from build123d import *

# Parameters (mm, degrees)
F1_DEPTH = 25.4
F2_SIZE  = 12.7
F3_T     = -2.54


with BuildPart() as f1:
    # F0 (on Top) → F1 (new body)
    with BuildSketch(Plane.XY):
        Polygon((4.5641, -68.949298), (57.429793, 38.427275), (-61.993893, 30.522022), align=None)
    extrude(amount=F1_DEPTH)

    # F2
    f2_edges = [f1.edges().sort_by_distance(p)[0] for p in [
        (30.996947, -15.261011, 25.4),
        (-28.714897, -19.213638, 25.4),
        (-2.28205, 34.474649, 25.4),
    ]]
    chamfer(f2_edges, length=F2_SIZE)

    # F3
    f3_openings = [f1.faces().sort_by_distance(p)[0] for p in [
        (0, 0, 25.4),
    ]]
    offset(amount=F3_T, openings=f3_openings)


solid = f1.part
Here's how the part is built. I have some questions about the finished solid (model axes, mm). A direction names the side the tool comes from. Coordinates: 2 decimals unless noted, no trailing zeros. Loops run counter-clockwise (first coordinate to the right, second up) from the corner with the lowest first, then second, coordinate; pieces in that order, holes last.
1. I need wall thicknesses on L1, parallel to Z at x = 2, y = -23.5; L2, parallel to X at y = -41, z = 14.75; L3, parallel to Y at x = -51.5, z = 2.75. Which ranges of each line are inside material? Lowest first, please.
2. For faces 1 (the flat face through (-0.879, 25.034, 18.62)), 2 (the flat face through (-1.021, 28.105, 19.139)), which set-ups out of +Z, -Z, +X, -X, +Y, -Y let a thin tool reach every point of the face, with its end or its side?
3. Imagine slicing it at D-D, the plane y = 10.5. Please give me the cut outline in (x, z), and give its area (3 significant figures).
4. Imagine slicing it at B-B, the plane x = 33. Please give me the cut outline in (y, z) (3 decimals), and give its area (3 significant figures).
5. For P1, Ø2, axis at x = -14.5, z = 4, coming from the -Y side; P2, Ø4, axis at x = 1.5, z = 4.5, coming from the +Y side; P3, Ø3, axis at x = -49.5, z = 13, coming from the +Y side, each with a flat end and sliding along its axis, tell me the tip position at first contact or that it passes through.
6. Imagine slicing it at A-A, the plane z = 10.25. Please give me the cut outline in (x, y), and give its area (3 significant figures).
7. Imagine slicing it at C-C, the plane y = -48. Please give me the cut outline in (x, z).
8. If we mould it in two halves opening along Y, with no side actions, what happens to faces 3 (the flat face through (-1.45, 34.53, 6.26)), 4 (the flat face through (-29.18, -18.52, 6.26)), 5 (the flat face through (-1.34, 31.99, 7.03))? For each: pulls with the +Y half, pulls with the -Y half, needs draft (parallel to the pull), parting line crosses it, or undercut.
Taken from the geometry:
1. L1: z = 0 to 2.54
1. L2: x = -11.67 to -7.35, 12.04 to 16.04
1. L3: y = 14.84 to 19.41, 28.67 to 31.22
2. face 1: none
2. face 2: +Z, -X, +Y
3. outline: (-48.6, 0) - (43.68, 0) - (43.68, 12.7) - (29.52, 25.4) - (25.52, 25.4) - (40.85, 11.65) - (40.85, 2.54) - (-45.54, 2.54) - (-45.54, 11.65) - (-28.99, 25.4) - (-33.32, 25.4) - (-48.6, 12.7) - close
3. area: 401 mm2
4. outline: (-11.193, 0) - (36.81, 0) - (36.81, 12.7) - (24.082, 25.4) - (17.56, 25.4) - (-11.193, 12.7) - close; hole (-5.442, 2.54) - (34.265, 2.54) - (34.265, 11.648) - (22.081, 23.805) - (-5.442, 11.648) - close
4. area: 353 mm2
5. P1: stops at y = -41.95
5. P2: stops at y = 34.86
5. P3: stops at y = 31.45
6. outline: (-61.99, 30.52) - (4.56, -68.95) - (57.43, 38.43) - close; hole (-57.44, 28.28) - (4.23, -63.88) - (53.21, 35.6) - close
6. area: 878 mm2
7. outline: (-9.45, 0) - (14.88, 0) - (14.88, 12.7) - (3.18, 23.2) - (-9.45, 12.7) - close; hole (-6.4, 2.54) - (12.05, 2.54) - (12.05, 11.65) - (3.18, 19.61) - (-6.4, 11.65) - close
8. face 3: pulls with the +Y half
8. face 4: pulls with the -Y half
8. face 5: undercut
